```python
from build123d import *

# Parameters (mm, degrees)
F0_R     = 15
F0_R_2   = 2.3
F0_R_3   = 1.65
F0_R_4   = 1.13
F1_DEPTH = 6
F2_DEPTH = 7
F3_R     = 2.3
F3_R_2   = 1.13
F4_DEPTH = 3


with BuildPart() as f1:
    # F0 (on Front) → F1 (new body)
    with BuildSketch(Plane.XZ):
        Circle(F0_R)
        Circle(F0_R_2, mode=Mode.SUBTRACT)
        Circle(F0_R_2)
        Circle(F0_R_3, mode=Mode.SUBTRACT)
        Circle(F0_R_3)
        Circle(F0_R_4, mode=Mode.SUBTRACT)
    extrude(amount=-F1_DEPTH)

    # F0 (on Front) → F2 (join)
    with BuildSketch(Plane.XZ):
        Circle(F0_R_3)
        Circle(F0_R_4, mode=Mode.SUBTRACT)
    extrude(amount=F2_DEPTH)

    # F3 (on face) → F4 (cut)
    with BuildSketch(Plane(origin=(0, 6, 0), x_dir=(-1, 0, 0), z_dir=(0, 1, 0))):
        Circle(F3_R)
        Circle(F3_R_2, mode=Mode.SUBTRACT)
    extrude(amount=-F4_DEPTH, mode=Mode.SUBTRACT)


solid = f1.part
```
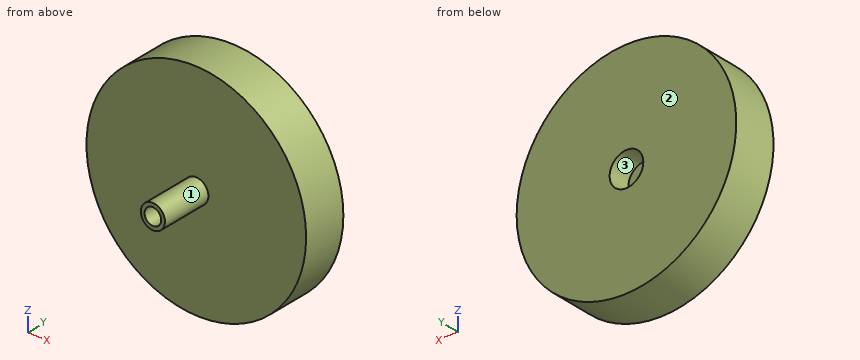
Work out the finished part from the listing and answer in its coordinate system (mm). Face numbers are marked on the shaded views. Give positions to 0.01 mm unless a question says otherwise; leave off trailing zeros. Loops run counter-clockwise (first coordinate to the right, second up) from the corner with the lowest first, then second, coordinate; pieces in that order, holes last. Notation, with made-up numbers: (-35.5, -3.75) - (-12.5, -3.75) arc R20 cw to (-12.5, 13.25) - close; hole circle Ø11 at (31.5, -22). An arc over 180 degrees is marked (long way). One line per question, with ' | ' between items.
(1) The part is cut by section C-C (y = 1). Write down the section's boundary in (x, z).
Recorded:
outline: circle Ø30 at (0, 0); hole circle Ø2.26 at (0, 0)
(2) Straight lines are drawn through the part: probe 1 along Z at (x, y) = (0, -2.75); probe 2 along Z at (x, y) = (0, 4.9); probe 3 along Y at (x, z) = (6.5, 9.25). For each, find the intervals that lie inside material, in ascending order.
Recorded:
probe 1: z = -1.65 to -1.13, 1.13 to 1.65 | probe 2: z = -15 to -2.3, 2.3 to 15 | probe 3: y = 0 to 6
(3) The part is cut by section A-A (x = 0). Write down the section's boundary in (y, z).
Recorded:
outline: (-7, -1.65) - (0, -1.65) - (0, -15) - (6, -15) - (6, -2.3) - (3, -2.3) - (3, -1.13) - (-7, -1.13) - close; (-7, 1.13) - (3, 1.13) - (3, 2.3) - (6, 2.3) - (6, 15) - (0, 15) - (0, 1.65) - (-7, 1.65) - close
(4) Each of these flat-tipped pins is pushed along its axis until it touches: pin 1 Ø3 at (y, z) = (-1, 4.5) entering from +X; pin 2 Ø12 at (x, z) = (-9, -3) entering from -Y; pin 3 Ø1.4 at (x, z) = (1, 0.5) entering from +Y. Where does it stop, or does it pass through?
Recorded:
pin 1: stops at x = 14.61 | pin 2: stops at y = 0 | pin 3: stops at y = 3
(5) The part is cut by section B-B (z = 0). Write down the section's boundary in (x, y).
Recorded:
outline: (-15, 0) - (-1.65, 0) - (-1.65, -7) - (-1.13, -7) - (-1.13, 3) - (-2.3, 3) - (-2.3, 6) - (-15, 6) - close; (1.13, -7) - (1.65, -7) - (1.65, 0) - (15, 0) - (15, 6) - (2.3, 6) - (2.3, 3) - (1.13, 3) - close
(6) The part is cut by section D-D (y = 3.5). Write down the section's boundary in (x, z), then the cut area to 3 significant figures.
Recorded:
outline: circle Ø30 at (0, 0); hole circle Ø4.6 at (0, 0) | area: 690 mm²
(7) The mould has two halves that part along Z. Classify the marked faces 1, 2 and 3: +Z half, -Z half, draft (parallel to the pull), parting line (faces both ways), or undercut.
Recorded:
face 1: parting line | face 2: draft | face 3: undercut
